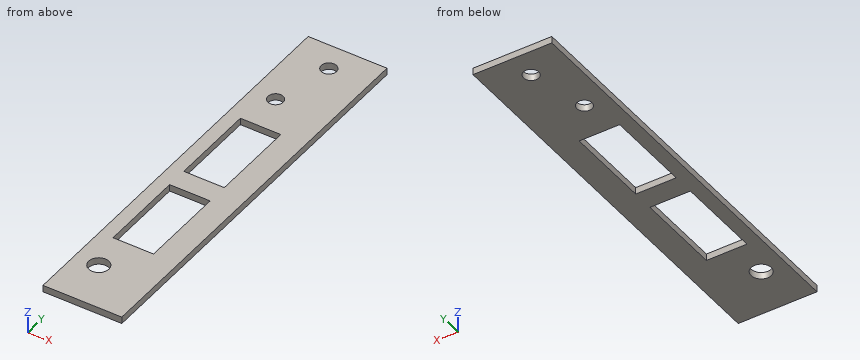
from build123d import *

# Parameters (mm, degrees)
SKETCH1_W          = 18.542
SKETCH1_H          = 95.25
EXTRUDE1_DEPTH     = 1.6002
SKETCH2_R          = 1.8034
CUT_EXTRUDE1_DEPTH = 1.6002
SKETCH3_R          = 1.778
SKETCH3_R_2        = 2.3749
CUT_EXTRUDE2_DEPTH = 2.54
SKETCH4_W          = 9.525
SKETCH4_H          = 20.32
FIBER_HOLES_DEPTH  = 2.54


with BuildPart() as part:
    # Sketch1 → Extrude1 (new body)
    with BuildSketch(Plane.XY):
        with Locations((9.271, -47.625)):
            Rectangle(SKETCH1_W, SKETCH1_H)
    extrude(amount=EXTRUDE1_DEPTH)

    # Sketch2 → Cut-Extrude1 (cut)
    with BuildSketch(Plane.XY.offset(1.6002)):
        with Locations((9.017, -6.35)):
            Circle(SKETCH2_R)
    extrude(amount=-CUT_EXTRUDE1_DEPTH, mode=Mode.SUBTRACT)

    # Sketch3 → Cut-Extrude2 (cut)
    with BuildSketch(Plane.XY.offset(1.6002)):
        with Locations((5.6388, -20.32)):
            Circle(SKETCH3_R)
        with Locations((5.6388, -83.82)):
            Circle(SKETCH3_R_2)
    extrude(amount=-CUT_EXTRUDE2_DEPTH, mode=Mode.SUBTRACT)

    # Sketch4 → Fiber Holes (cut)
    with BuildSketch(Plane.XY.offset(1.6002)):
        with Locations((7.9375, -39.37)):
            Rectangle(SKETCH4_W, SKETCH4_H)
        with Locations((7.9375, -64.77)):
            Rectangle(SKETCH4_W, SKETCH4_H)
    extrude(amount=-FIBER_HOLES_DEPTH, mode=Mode.SUBTRACT)


solid = part.part
Work out the finished part from the listing and answer in its coordinate system (mm). Round coordinates to 2 decimals unless told otherwise and drop trailing zeros. Loops run counter-clockwise (first coordinate to the right, second up) from the corner with the lowest first, then second, coordinate; pieces in that order, holes last. Notation, with made-up numbers: (57.5, 84) - (80.5, 84) arc R23 ccw to (80.5, 112) - close; hole circle Ø9 at (31.5, 87.25). An arc over 180 degrees is marked (long way). One line per item, written item: value.
Q1. Find section C-C on x = 6.25. Give the vertices of the cut face in (y, z), and give its area (3 significant figures).
Check values:
outline: (-95.25, 0) - (-86.11, 0) - (-86.11, 1.6) - (-95.25, 1.6) - close; (-81.53, 0) - (-74.93, 0) - (-74.93, 1.6) - (-81.53, 1.6) - close; (-54.61, 0) - (-49.53, 0) - (-49.53, 1.6) - (-54.61, 1.6) - close; (-29.21, 0) - (-21.99, 0) - (-21.99, 1.6) - (-29.21, 1.6) - close; (-18.65, 0) - (0, 0) - (0, 1.6) - (-18.65, 1.6) - close
area: 74.7 mm2
Q2. Find section B-B on z = 0.85. Give the vertices of the cut face in (x, y) (3 decimals), and give its area (3 significant figures).
Check values:
outline: (0, -95.25) - (18.542, -95.25) - (18.542, 0) - (0, 0) - close; hole (3.175, -74.93) - (12.7, -74.93) - (12.7, -54.61) - (3.175, -54.61) - close; hole (3.175, -49.53) - (12.7, -49.53) - (12.7, -29.21) - (3.175, -29.21) - close; hole circle Ø4.75 at (5.639, -83.82); hole circle Ø3.556 at (5.639, -20.32); hole circle Ø3.607 at (9.017, -6.35)
area: 1,340 mm2
Q3. Straight lines are drawn through the part: probe 1 along Y at (x, z) = (12.5, 1.5); probe 2 along X at (y, z) = (-65, 0.7) (3 decimals); probe 3 along X at (y, z) = (-7, 1.25). For each, find the intervals that lie inside material, in ascending order.
Check values:
probe 1: -95.25 to -74.93, -54.61 to -49.53, -29.21 to 0
probe 2: 0 to 3.175, 12.7 to 18.542
probe 3: 0 to 7.33, 10.7 to 18.54
Q4. Find section A-A on y = -20.32. Give the vertices of the cut face in (x, z).
Check values:
outline: (0, 0) - (3.86, 0) - (3.86, 1.6) - (0, 1.6) - close; (7.42, 0) - (18.54, 0) - (18.54, 1.6) - (7.42, 1.6) - close
Q5. Find section D-D on y = -44.5. Give the vertices of the cut face in (x, z) (3 decimals), and give its area (3 significant figures).
Check values:
outline: (0, 0) - (3.175, 0) - (3.175, 1.6) - (0, 1.6) - close; (12.7, 0) - (18.542, 0) - (18.542, 1.6) - (12.7, 1.6) - close
area: 14.4 mm2
